Read the model definition and answer for the solid it produces. Units are mm, in the model's axes. Round coordinates to 2 decimals unless told otherwise and drop trailing zeros. Loops run counter-clockwise (first coordinate to the right, second up) from the corner with the lowest first, then second, coordinate; pieces in that order, holes last. Notation, with made-up numbers: (-16.75, -39.75) - (1.25, -39.75) arc R9 cw to (1.25, -24.75) - close; hole circle Ø5 at (11.25, -15.75). An arc over 180 degrees is marked (long way). Use CSV: the item, a comma, the result in double quotes. Start each with the question number.
1. Find section B-B (x = -967.5). Give the vertices of the cut face in (y, z), and give its area (3 significant figures).
2. Given pin 1 Ø5.5 at (x, z) = (-1030.5, 304.5) entering from -Y; pin 2 Ø5.5 at (y, z) = (168, 305.5) entering from -X; pin 3 Ø5 at (x, y) = (-474, 66.5) entering from -Z, each flat-ended and moving along its own axis, determine where each tip first touches the part or whether it passes through.
3. Find section A-A (z = 304.75). State how many separate pieces and enclosed holes the cut face has, and give its area (3 significant figures).
4. Consider line 1 along X through (y, z) = (125, 309); line 2 along X through (y, z) = (161.5, 309) (3 decimals); line 3 along Y through (x, z) = (-121.5, 298.25). Determine where each line is inside the solid, lowest interval first.
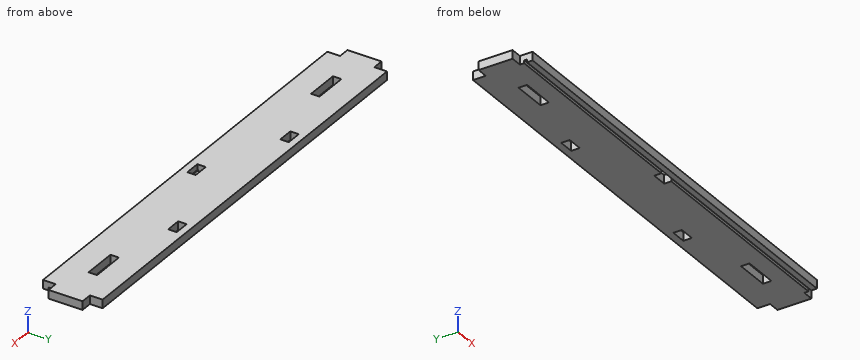
from build123d import *

# Parameters (mm, degrees)
SKETCH1_W           = 19.05
SKETCH1_H           = 133.35
BOSS_EXTRUDE1_DEPTH = 1041.4
SKETCH2_W           = 76.2
SKETCH2_H           = 19.05
SKETCH2_W_2         = 34.925
SKETCH2_W_3         = 25.4
SKETCH2_H_2         = 28.575
CUT_EXTRUDE1_DEPTH  = 1058.779929099
SKETCH3_W           = 6.35
SKETCH3_H           = 6.35
CUT_EXTRUDE2_DEPTH  = 1103.515918102


with BuildPart() as part:
    # Sketch1 → Boss-Extrude1 (new body)
    with BuildSketch(Plane(origin=(0, 0, 0), x_dir=(0, 0, -1), z_dir=(1, 0, 0))):
        with Locations((-301.932659665, 117.774223108)):
            Rectangle(SKETCH1_W, SKETCH1_H)
    extrude(amount=-BOSS_EXTRUDE1_DEPTH)

    # Sketch2 → Cut-Extrude1 (cut, through all)
    with BuildSketch(Plane.XY.offset(311.457659665)):
        with Locations((-908.05, 117.774223108)):
            Rectangle(SKETCH2_W, SKETCH2_H)
        with Locations((-133.35, 117.774223108)):
            Rectangle(SKETCH2_W, SKETCH2_H)
        with Locations((-325.4375, 159.036523108)):
            Rectangle(SKETCH2_W_2, SKETCH2_H)
        with Locations((-715.9625, 159.036523108)):
            Rectangle(SKETCH2_W_2, SKETCH2_H)
        with Locations((-12.7, 170.161723108)):
            Rectangle(SKETCH2_W_3, SKETCH2_H_2)
        with Locations((-1028.7, 170.161723108)):
            Rectangle(SKETCH2_W_3, SKETCH2_H_2)
        with Locations((-520.7, 76.499223108)):
            Rectangle(SKETCH2_W_2, SKETCH2_H)
        with Locations((-1028.7, 65.386723108)):
            Rectangle(SKETCH2_W_3, SKETCH2_H_2)
        with Locations((-12.7, 65.386723108)):
            Rectangle(SKETCH2_W_3, SKETCH2_H_2)
    extrude(amount=-CUT_EXTRUDE1_DEPTH, mode=Mode.SUBTRACT)

    # Sketch3 → Cut-Extrude2 (cut, through all)
    with BuildSketch(Plane.ZY.offset(1041.4)):
        with Locations((295.582659665, 66.974223108)):
            Rectangle(SKETCH3_W, SKETCH3_H)
    extrude(amount=-CUT_EXTRUDE2_DEPTH, mode=Mode.SUBTRACT)


solid = part.part
Filled sheet:
1,outline,"(51.1, 292.41) - (63.8, 292.41) - (63.8, 298.76) - (70.15, 298.76) - (70.15, 292.41) - (184.45, 292.41) - (184.45, 311.46) - (51.1, 311.46) - close"
1,area,"2,500 mm²"
2,pin 1,"stops at y = 79.67"
2,pin 2,"stops at x = -1016"
2,pin 3,"stops at z = 298.76"
3,separate pieces,"1"
3,enclosed holes,"5"
3,area,"131,000 mm²"
4,line 1,"x = -1041.4 to -946.15, -869.95 to -171.45, -95.25 to 0"
4,line 2,"x = -1016 to -733.425, -698.5 to -342.9, -307.975 to -25.4"
4,line 3,"y = 51.1 to 63.8, 70.15 to 108.25, 127.3 to 184.45"
